Input: part model. Units: mm. Frame: model coordinates. Give positions to 0.01 mm unless a question says otherwise; leave off trailing zeros. Loops run counter-clockwise (first coordinate to the right, second up) from the corner with the lowest first, then second, coordinate; pieces in that order, holes last. Notation, with made-up numbers: M 65,78 L 113,78 A21 ccw 113,101 Z; hole C -22.75,86 d10. An arc over 180 degrees is marked long. Use a Markdown table: item, result. Add a question column.
from build123d import *

# Parameters (mm, degrees)
SKETCH1_R           = 12
BOSS_EXTRUDE1_DEPTH = 11
CHAMFER1_SIZE       = 2
SKETCH2_R           = 2.6
CUT_EXTRUDE1_DEPTH  = 11


with BuildPart() as part:
    # Sketch1 → Boss-Extrude1 (new body)
    with BuildSketch(Plane.XY):
        Circle(SKETCH1_R)
    extrude(amount=BOSS_EXTRUDE1_DEPTH)

    # Chamfer1
    chamfer1_edges = [part.edges().sort_by_distance(p)[0] for p in [
        (-12, 0, 0),
        (-12, 0, 11),
    ]]
    chamfer(chamfer1_edges, length=CHAMFER1_SIZE)

    # Sketch2 → Cut-Extrude1 (cut)
    with BuildSketch(Plane.XY.offset(11)):
        Circle(SKETCH2_R)
    extrude(amount=-CUT_EXTRUDE1_DEPTH, mode=Mode.SUBTRACT)


solid = part.part
1) Section query A-A, the plane x = 0. Return the cut outline in (y, z), and give its area (3 significant figures).
2) Pull-direction query (X, two-part tool) for faces 1 (the flat face through (2, -2, 0)), 2 (the cylindrical face through (-11.99, 0.53, 5.45)), 3 (the cylindrical face through (-0.338, 2.578, 5.577)); classes: pulls with the +X half, pulls with the -X half, needs draft (parallel to the pull), parting line crosses it, or undercut.
3) Contact query for flat-ended pins moving along their axis: P1, Ø6, axis at x = -5.5, z = 2, coming from the -Y side; P2, Ø4, axis at x = -3.5, z = 9.5, coming from the +Y side; P3, Ø1.5, axis at y = -7.5, z = 7, coming from the +X side. Output: stop coordinate, or through.
4) Section query C-C, the plane z = 4.5. Return the cut outline in (x, y).
5) Ray query, line 1 (Y direction, x = 0, z = 8); line 2 (X direction, y = -0.5, z = 9); line 3 (X direction, y = 9.5, z = 1). Return the intervals inside material, ascending. Write a range as [from, to].
Entries:
| question | item | result |
|---|---|---|
| 1 | outline | M -12,2 L -10,0 L -2.6,0 L -2.6,11 L -10,11 L -12,9 Z; M 2.6,0 L 10,0 L 12,2 L 12,9 L 10,11 L 2.6,11 Z |
| 1 | area | 199 mm² |
| 2 | face 1 | needs draft |
| 2 | face 2 | parting line crosses it |
| 2 | face 3 | undercut |
| 3 | P1 | stops at y = -11.74 |
| 3 | P2 | stops at y = 11.9 |
| 3 | P3 | stops at x = 9.92 |
| 4 | outline | C 0,0 d24; hole C 0,0 d5.2 |
| 5 | line 1 | y = [-12, -2.6], [2.6, 12] |
| 5 | line 2 | x = [-11.99, -2.55], [2.55, 11.99] |
| 5 | line 3 | x = [-5.55, 5.55] |
